Autodesk Fusion 360 part; units mm, degrees
sketch "Sketch1" plane through (0, 0, 0) normal (0, 0, 1) x (1, 0, 0)
  line L0 (4, 4) -> (32, 4)
  line L1 (32, 4) -> (32, 42)
  line L2 (32, 42) -> (4, 42)
  line L3 (4, 42) -> (4, 4)
  line L4 (0, 0) -> (36, 0)
  line L5 (36, 0) -> (36, 46)
  line L6 (36, 46) -> (0, 46)
  line L7 (0, 46) -> (0, 0)
  circle A0 centre (18, 23) radius 14
  dimension "d1" = 28
  dimension "d2" = 38
  dimension "d3" = 36
  dimension "d4" = 46
  dimension "d5" = 4
  dimension "d6" = 4
extrude "Extrude1" add sketch "Sketch1" along normal blind 23
extrude "Extrude2" add sketch "Sketch1" along normal blind 3 contours L0 L1 L3 A0 | L1 L2 L3 A0 | A0
extrude "Extrude3" add sketch "Sketch1" along normal blind 1 from surface at 22 contours L0 L1 L3 A0 | L1 L2 L3 A0
sketch "Sketch2" plane through (0, 0, 0) normal (0, -1, 0) x (1, 0, 0)
  line L0 (0, 0) -> (36, 0)
  line L1 (36, 0) -> (36, 23)
  line L2 (36, 23) -> (0, 23)
  line L3 (0, 23) -> (0, 0)
  line L4 (10, 12) -> (28, 12)
  line L5 (28, 12) -> (28, 5)
  line L6 (28, 5) -> (10, 5)
  line L7 (10, 5) -> (10, 12)
  line L8 (0, 0) -> (36, 0)
  dimension "d14" = 18
  dimension "d15" = 7
  dimension "d16" = 5
extrude "Extrude4" cut sketch "Sketch2" against normal blind 4 contours L4 L5 L6 L7
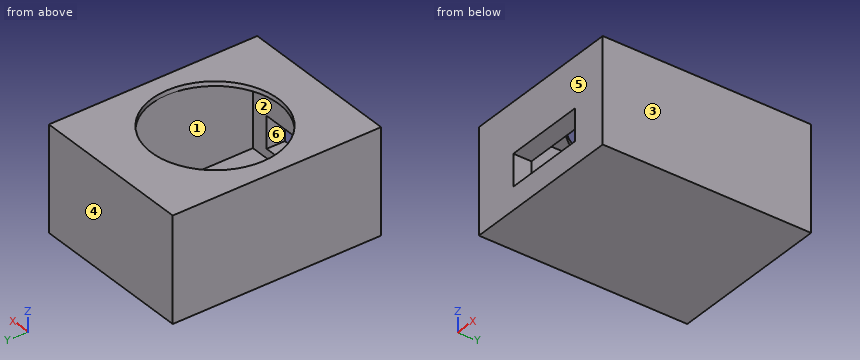
Source: CAD feature listing. Evaluate the final solid. Frame: model axes, mm. Face numbers are marked on the shaded views. A direction names the side the tool comes from. Round coordinates to 2 decimals unless told otherwise and drop trailing zeros. Write each loop counter-clockwise with the first axis right and the second up, starting at its lowest first coordinate (ties: lowest second). Pieces come first, ordered by that corner, then holes. Notation, with made-up numbers: (-39.75, 27.25) - (4.25, 27.25) arc R24 cw to (4.25, 41.25) - close; hole circle Ø4 at (10.5, -28). An arc over 180 degrees is marked (long way). Use CSV: the item, a comma, the result in double quotes. Start each with the question number.
(1) First-contact query: pin 1 Ø14 at (x, y) = (13, 21.5) entering from +Z. Flat tip, straight axial feed; report the tip coordinate or a pass-through.
(2) Material intervals for probe 1 along Z at (x, y) = (4.5, 27); probe 2 along Y at (x, z) = (12, 20.5); probe 3 along X at (y, z) = (23, 22.75), sorted ascending. Write a range as [from, to].
(3) Cut plane C-C, the plane y = 3. Return loops of the section in (x, z).
(4) Cut plane A-A, the plane z = 16.75. Return loops of the section in (x, y), and give its area (3 significant figures).
(5) Set-up query: the marked faces 5 and 6. Return all of +Z, -Z, +X, -X, +Y, -Y with unobstructed straight access to the full face (end or side cutting, diameter ignored); none if empty.
(6) Cut plane B-B, the plane x = 23. Return loops of the section in (y, z).
(7) Mould query, pull axis X, two halves, no side actions, for the marked faces 1, 2, 3 and 4. Classes: pulls with the +X half, pulls with the -X half, needs draft (parallel to the pull), parting line crosses it, or undercut.
(8) Cut plane D-D, the plane z = 8.5. Return loops of the section in (x, y), and give its area (3 significant figures).
Geometry says:
1,pin 1,"z = 3"
2,probe 1,"[0, 3], [22, 23]"
2,probe 2,"[0, 4], [42, 46]"
2,probe 3,"[0, 4], [32, 36]"
3,outline,"(0, 0) - (36, 0) - (36, 23) - (0, 23) - close; hole (10, 5) - (28, 5) - (28, 12) - (10, 12) - close"
4,outline,"(0, 0) - (36, 0) - (36, 46) - (0, 46) - close; hole (4, 4) - (32, 4) - (32, 42) - (4, 42) - close"
4,area,"592 mm²"
5,face 5,"+Z, -Z, +X, -X, -Y"
5,face 6,"-Y"
6,outline,"(0, 0) - (46, 0) - (46, 23) - (36.08, 23) - (36.08, 22) - (42, 22) - (42, 3) - (4, 3) - (4, 5) - (0, 5) - close; (0, 12) - (4, 12) - (4, 22) - (9.92, 22) - (9.92, 23) - (0, 23) - close"
7,face 1,"undercut"
7,face 2,"undercut"
7,face 3,"pulls with the +X half"
7,face 4,"needs draft"
8,outline,"(0, 0) - (10, 0) - (10, 4) - (4, 4) - (4, 42) - (32, 42) - (32, 4) - (28, 4) - (28, 0) - (36, 0) - (36, 46) - (0, 46) - close"
8,area,"520 mm²"
